from build123d import *

# Parameters (mm, degrees)
BOSS_EXTRUDE1_DEPTH = 15.24
BOSS_EXTRUDE2_DEPTH = 1.27
CIRPATTERN1_COUNT   = 3
SKETCH4_R           = 31.75
SKETCH4_R_2         = 19.05
BOSS_EXTRUDE3_DEPTH = 2.54
SKETCH5_R           = 19.05
CUT_EXTRUDE1_DEPTH  = 16.24


with BuildPart() as part:
    # Sketch2 → Boss-Extrude1 (new body)
    with BuildSketch(Plane(origin=(0, 0, 0), x_dir=(1, 0, 0), z_dir=(0, 1, 0))):
        Polygon((-1.27, 0), (0, 2.199704526), (1.27, 0), align=None)
    extrude(amount=BOSS_EXTRUDE1_DEPTH)

    # Sketch3 → Boss-Extrude2 (add, symmetric)
    with BuildSketch(Plane(origin=(0, 0, 0), x_dir=(0, 0, -1), z_dir=(1, 0, 0))):
        Polygon((0, 15.24), (-63.627, 15.24), (0, 0), align=None)
    boss_extrude2 = extrude(amount=BOSS_EXTRUDE2_DEPTH, both=True)

    # CirPattern1: Boss-Extrude2 ×3 about axis
    cirpattern1_axis = Axis((0, 0, -0.733234842), (0, 1, 0))
    for i in range(1, CIRPATTERN1_COUNT):
        add(boss_extrude2.rotate(cirpattern1_axis, i * 360 / CIRPATTERN1_COUNT))

    # Sketch4 → Boss-Extrude3 (add)
    with BuildSketch(Plane(origin=(0, 15.24, 0), x_dir=(1, 0, 0), z_dir=(0, 1, 0))):
        Circle(SKETCH4_R)
        Circle(SKETCH4_R_2, mode=Mode.SUBTRACT)
    extrude(amount=-BOSS_EXTRUDE3_DEPTH)

    # Sketch5 → Cut-Extrude1 (cut, through all)
    with BuildSketch(Plane(origin=(0, 15.24, 0), x_dir=(1, 0, 0), z_dir=(0, 1, 0))):
        Circle(SKETCH5_R)
    extrude(amount=-CUT_EXTRUDE1_DEPTH, mode=Mode.SUBTRACT)


solid = part.part
Design review of the part built by this model. Coordinates are the model's own, in mm. A direction names the side the tool comes from. Round coordinates to 2 decimals unless told otherwise and drop trailing zeros. Write each loop counter-clockwise with the first axis right and the second up, starting at its lowest first coordinate (ties: lowest second). Pieces come first, ordered by that corner, then holes. Notation, with made-up numbers: (8, -38) -> (60, -38) arc R25 cw to (60, 0) -> close; hole circle Ø10 at (-19.75, 71.5). An arc over 180 degrees is marked (long way). One line per item, written item: value. Start each with the question number.
Q1. Add section A-A (z = 0). Give the boundary of the cut face in (x, y).
Q2. Add section B-B (x = 0). Give the boundary of the cut face in (y, z), then the cut area to 3 significant figures.
Q3. The part is to be moulded in two halves that separate along X. For faces 5 (the face through (-32.47, 11.061, -18.013)), 6 (the face through (-13, 15.24, 15)), 7 (the face through (15.81, 13.44, -10.63)), 8 (the face through (32.47, 11.061, -18.013)), say which applies: pulls with the +X half, pulls with the -X half, needs draft (parallel to the pull), parting line crosses it, or undercut.
Q4. Add section C-C (y = 6.75). Give the boundary of the cut face in (x, z).
Q5. Tool access review of faces 1 (the face through (1.27, 11, 37)), 2 (the face through (0.02, 9.97, 41.63)), 3 (the face through (31.16, 11.05, -20.19)), 4 (the face through (-20, 12.7, 13)): name each direction out of +Z, -Z, +X, -X, +Y, -Y from which nothing blocks a thin tool from reaching the whole face with its end or side.
Q6. Add section D-D (x = -21). Give the boundary of the cut face in (y, z), then the cut area to 3 significant figures.
Q7. Insertion check: P1, Ø4, axis at x = -33, y = 10, coming from the -Z side; P2, Ø6, axis at x = -5.5, z = -20, coming from the -Y side; P3, Ø6, axis at y = 8, z = 28.5, coming from the -X side; P4, Ø10, axis at x = 10.5, z = -8.5, coming from the +Y side. Each pin has a flat end and moves straight along its axis. Give the tip position at first contact, or say it passes through.
Q8. To check wall thickness, follow probe 1 along X at (y, z) = (13, 0); probe 2 along X at (y, z) = (12, -16.5); probe 3 along Z at (x, y) = (-4.5, 14.5). State the ranges of each line that lie inside material, in increasing order.
Response:
1. outline: (-31.75, 12.7) -> (-19.05, 12.7) -> (-19.05, 15.24) -> (-31.75, 15.24) -> close; (19.05, 12.7) -> (31.75, 12.7) -> (31.75, 15.24) -> (19.05, 15.24) -> close
2. outline: (4.56, 19.05) -> (15.24, 19.05) -> (15.24, 63.63) -> close; (12.7, -31.75) -> (15.24, -31.75) -> (15.24, -19.05) -> (12.7, -19.05) -> close
2. area: 270 mm^2
3. face 5: pulls with the -X half
3. face 6: needs draft
3. face 7: undercut
3. face 8: pulls with the +X half
4. outline: (-25.68, -14.09) -> (-24.41, -16.29) -> (-15.46, -11.13) arc R19.05 cw to (-16.81, -8.97) -> close; (-1.27, 19.01) arc R19.05 cw to (1.27, 19.01) -> (1.27, 28.18) -> (-1.27, 28.18) -> close; (15.46, -11.13) -> (24.41, -16.29) -> (25.68, -14.09) -> (16.81, -8.97) arc R19.05 cw to start
5. face 1: +Z, +X, -Y
5. face 2: +Z, +X, -X, -Y
5. face 3: -Z, -Y
5. face 4: +Z, -X, -Y
6. outline: (5.46, -11.39) -> (5.81, -14.32) -> (12.7, -14.32) -> (12.7, -23.81) -> (15.24, -23.81) -> (15.24, 23.81) -> (12.7, 23.81) -> (12.7, -11.39) -> close
6. area: 142 mm^2
7. P1: stops at z = -22.41
7. P2: stops at y = 12.7
7. P3: stops at x = -1.27
7. P4: passes through
8. probe 1: x = -31.75 to -19.05, 19.05 to 31.75
8. probe 2: x = -29.85 to -24.77, 24.77 to 29.85
8. probe 3: z = -31.43 to -18.51, 18.51 to 31.43
